from build123d import *

# Parameters (mm, degrees)
BOSS_EXTRUDE1_DEPTH     = 3
SKETCH2_R               = 10
SKETCH2_W               = 15
SKETCH2_H               = 20
CUT_EXTRUDE4_DEPTH      = 7
CUT_EXTRUDE4_DEPTH_BACK = 3
SKETCH6_W               = 65
SKETCH6_H               = 35
BOSS_EXTRUDE5_DEPTH     = 1.3


with BuildPart() as part:
    # Sketch1 → Boss-Extrude1 (new body)
    with BuildSketch(Plane(origin=(0, 0, 0), x_dir=(1, 0, 0), z_dir=(0, 1, 0))):
        with BuildLine():
            Line((5, 0), (70, 0))
            ThreePointArc((70, 0), (73.535533906, 1.464466094), (75, 5))
            Line((75, 5), (75, 85))
            ThreePointArc((75, 85), (73.535533906, 88.535533906), (70, 90))
            Line((70, 90), (5, 90))
            ThreePointArc((5, 90), (1.464466094, 88.535533906), (0, 85))
            Line((0, 85), (0, 5))
            ThreePointArc((0, 5), (1.464466094, 1.464466094), (5, 0))
        make_face()
    extrude(amount=BOSS_EXTRUDE1_DEPTH)

    # Sketch2 → Cut-Extrude4 (cut, two sides)
    with BuildSketch(Plane(origin=(0, 0, 0), x_dir=(1, 0, 0), z_dir=(0, 1, 0))) as cut_extrude4_sk:
        with Locations((47, 75)):
            Circle(SKETCH2_R)
        with BuildLine():
            Line((8, 5.5), (67, 5.5))
            ThreePointArc((67, 5.5), (69.121320344, 6.378679656), (70, 8.5))
            Line((70, 8.5), (70, 37.5))
            ThreePointArc((70, 37.5), (69.121320344, 39.621320344), (67, 40.5))
            Line((67, 40.5), (8, 40.5))
            ThreePointArc((8, 40.5), (5.878679656, 39.621320344), (5, 37.5))
            Line((5, 37.5), (5, 8.5))
            ThreePointArc((5, 8.5), (5.878679656, 6.378679656), (8, 5.5))
        make_face()
        with Locations((10, 53.5)):
            Rectangle(SKETCH2_W, SKETCH2_H)
    extrude(amount=CUT_EXTRUDE4_DEPTH, mode=Mode.SUBTRACT)
    extrude(cut_extrude4_sk.sketch, amount=-CUT_EXTRUDE4_DEPTH_BACK, mode=Mode.SUBTRACT)

    # Sketch6 → Boss-Extrude5 (add)
    with BuildSketch(Plane(origin=(0, 0, 0), x_dir=(1, 0, 0), z_dir=(0, 1, 0))):
        with Locations((37.5, 23)):
            Rectangle(SKETCH6_W, SKETCH6_H)
        with BuildLine():
            Line((9, 38.5), (66, 38.5))
            ThreePointArc((66, 38.5), (67.414213562, 37.914213562), (68, 36.5))
            Line((68, 36.5), (68, 9.5))
            ThreePointArc((68, 9.5), (67.414213562, 8.085786438), (66, 7.5))
            Line((66, 7.5), (9, 7.5))
            ThreePointArc((9, 7.5), (7.585786438, 8.085786438), (7, 9.5))
            Line((7, 9.5), (7, 36.5))
            ThreePointArc((7, 36.5), (7.585786438, 37.914213562), (9, 38.5))
        make_face(mode=Mode.SUBTRACT)
    extrude(amount=BOSS_EXTRUDE5_DEPTH)


solid = part.part
Geometry check sheet. Reference: the model listing, model coordinates, mm. A direction names the side the tool comes from. Give positions to 0.01 mm unless a question says otherwise; leave off trailing zeros. Write each loop counter-clockwise with the first axis right and the second up, starting at its lowest first coordinate (ties: lowest second). Pieces come first, ordered by that corner, then holes.
1) Cross-section at C-C (y = 1.95). Record the boundary of the cut face in (x, z).
Values follow:
outline: (0, -85) arc R5 ccw to (5, -90) - (70, -90) arc R5 ccw to (75, -85) - (75, -5) arc R5 ccw to (70, 0) - (5, 0) arc R5 ccw to (0, -5) - close; hole (2.5, -63.5) - (17.5, -63.5) - (17.5, -43.5) - (2.5, -43.5) - close; hole (5, -37.5) arc R3 ccw to (8, -40.5) - (67, -40.5) arc R3 ccw to (70, -37.5) - (70, -8.5) arc R3 ccw to (67, -5.5) - (8, -5.5) arc R3 ccw to (5, -8.5) - close; hole circle Ø20 at (47, -75)
2) Cross-section at B-B (z = -75). Record the boundary of the cut face in (x, y).
Values follow:
outline: (0, 0) - (37, 0) - (37, 3) - (0, 3) - close; (57, 0) - (75, 0) - (75, 3) - (57, 3) - close
3) Set-up check for faces 4 (the face through (73, 1, -1)), 5 (the face through (7.6, 0.64, -8.07)), 6 (the face through (37, 1.3, -39)): record each of +Z, -Z, +X, -X, +Y, -Y from which the full face is reachable in a straight line by a thin tool's end or side.
Values follow:
face 4: +Z, +X, +Y, -Y
face 5: +Y, -Y
face 6: +Y
4) Cross-section at D-D (x = 32). Record the boundary of the cut face in (y, z), plus the area to 3 significant figures.
Values follow:
outline: (0, -90) - (3, -90) - (3, -40.5) - (1.3, -40.5) - (1.3, -38.5) - (0, -38.5) - close; (0, -7.5) - (1.3, -7.5) - (1.3, -5.5) - (3, -5.5) - (3, 0) - (0, 0) - close
area: 170 mm2
5) Cross-section at A-A (x = 47). Record the boundary of the cut face in (y, z), plus the area to 3 significant figures.
Values follow:
outline: (0, -90) - (3, -90) - (3, -85) - (0, -85) - close; (0, -65) - (3, -65) - (3, -40.5) - (1.3, -40.5) - (1.3, -38.5) - (0, -38.5) - close; (0, -7.5) - (1.3, -7.5) - (1.3, -5.5) - (3, -5.5) - (3, 0) - (0, 0) - close
area: 110 mm2
6) Release check for a two-part mould opening along Z. For faces 1 (the face through (5.86, 2.14, -6.4)), 2 (the face through (38, 1, -90)), 3 (the face through (37, 0, -56)) record: released by +Z, released by -Z, zero draft, split by the parting line, or undercut.
Values follow:
face 1: undercut
face 2: released by -Z
face 3: zero draft
7) Thickness scan on line 1 (Z direction, x = 47, y = 1.35); line 2 (Z direction, x = 9, y = 1.8); line 3 (X direction, y = 0.65, z = -75). Record the ranges inside material, lowest first.
Values follow:
line 1: z = -90 to -85, -65 to -40.5, -5.5 to 0
line 2: z = -90 to -63.5, -43.5 to -40.5, -5.5 to 0
line 3: x = 0 to 37, 57 to 75
